Check sheet for the modelled part. Datum: model origin and axes. Units: mm. Face numbers are marked on the shaded views. Give positions to 0.01 mm unless a question says otherwise; leave off trailing zeros. Order: outer loops, then holes, each group sorted by start corner. A loop starts at its lowest first (then second) coordinate and runs counter-clockwise, first axis right, second up. Notation, with made-up numbers: M 6.25,73.5 L 32.25,73.5 A13 ccw 32.25,95.5 Z; hole C 17,50 d1. An arc over 180 degrees is marked long. Return JSON: item names as keys, results as strings. Group by question number.
from build123d import *

# Parameters (mm, degrees)
SKETCH_1_R          = 325
EXTRUDE_1_DEPTH     = 255
CUT_EXTRUDE_2_DEPTH = 255
CUT_EXTRUDE_3_DEPTH = 255
CUT_EXTRUDE_5_DEPTH = 255
CUT_EXTRUDE_6_DEPTH = 255


with BuildPart() as part:
    # 草图1 → 凸台-拉伸1 (new body)
    with BuildSketch(Plane.XY):
        Circle(SKETCH_1_R)
    extrude(amount=EXTRUDE_1_DEPTH)

    # 草图2 → 切除-拉伸2 (cut)
    with BuildSketch(Plane.XY):
        with BuildLine():
            Line((51.961524227, 30), (250, 30))
            ThreePointArc((250, 30), (185.563491861, 185.563491861), (30, 250))
            Line((30, 250), (30, 51.961524227))
            ThreePointArc((30, 51.961524227), (42.426406871, 42.426406871), (51.961524227, 30))
        make_face()
    extrude(amount=CUT_EXTRUDE_2_DEPTH, mode=Mode.SUBTRACT)

    # 草图3 → 切除-拉伸3 (cut)
    with BuildSketch(Plane.XY):
        with BuildLine():
            Line((-30, 250), (-30, 51.961524227))
            ThreePointArc((-30, 51.961524227), (-42.426406871, 42.426406871), (-51.961524227, 30))
            Line((-51.961524227, 30), (-250, 30))
            ThreePointArc((-250, 30), (-185.563491861, 185.563491861), (-30, 250))
        make_face()
    extrude(amount=CUT_EXTRUDE_3_DEPTH, mode=Mode.SUBTRACT)

    # 草图7 → 切除-拉伸5 (cut)
    with BuildSketch(Plane.XY):
        with BuildLine():
            Line((-30, -51.961524227), (-30, -250))
            ThreePointArc((-30, -250), (-185.563491861, -185.563491861), (-250, -30))
            Line((-250, -30), (-51.961524227, -30))
            ThreePointArc((-51.961524227, -30), (-42.426406871, -42.426406871), (-30, -51.961524227))
        make_face()
    extrude(amount=CUT_EXTRUDE_5_DEPTH, mode=Mode.SUBTRACT)

    # 草图8 → 切除-拉伸6 (cut)
    with BuildSketch(Plane.XY):
        with BuildLine():
            Line((30, -30), (30, -250))
            ThreePointArc((30, -250), (185.563491861, -185.563491861), (250, -30))
            Line((250, -30), (30, -30))
        make_face()
    extrude(amount=CUT_EXTRUDE_6_DEPTH, mode=Mode.SUBTRACT)


solid = part.part
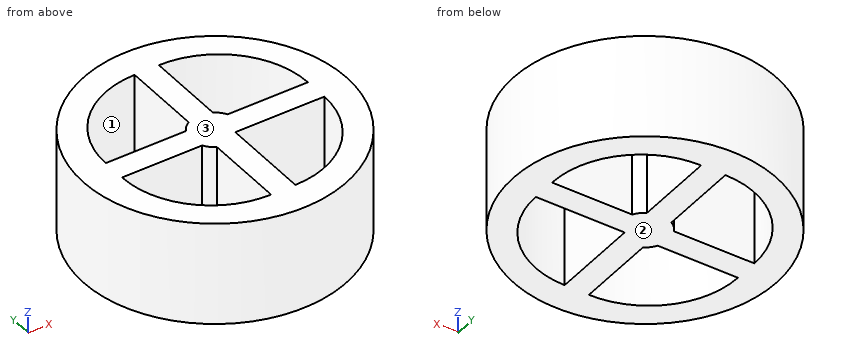
1) Sectioned sample at D-D on x = 266. Record the boundary of the cut face in (y, z).
2) Sectioned sample at A-A on y = -122.5. Record the boundary of the cut face in (x, z), then the cut area to 3 significant figures.
3) Release check for a two-part mould opening along Z. For the marked faces 1, 2 and 3 record: released by +Z, released by -Z, zero draft, split by the parting line, or undercut.
4) Sectioned sample at B-B on z = 91. Record the boundary of the cut face in (x, y), then the cut area to 3 significant figures.
5) Depth check by flat-ended pin: P1, Ø10, axis at x = -81, z = 30.5, coming from the -Y side; P2, Ø4, axis at x = 24, z = 84.5, coming from the -Y side; P3, Ø1.5, axis at y = 70, z = 72.5, coming from the +X side. Enter the tip coordinate at first touch or a pass-through.
6) Material ranges on line 1 along X through (y, z) = (-168.5, 104.5); line 2 along Y through (x, z) = (205, 216.5); line 3 along X through (y, z) = (-165, 18), recorded low to high.
7) Sectioned sample at C-C on x = 112.5. Record the boundary of the cut face in (y, z), then the cut area to 3 significant figures.
Reply:
{
 "1": {"outline": "M -186.73,0 L 186.73,0 L 186.73,255 L -186.73,255 Z"},
 "2": {"outline": "M -301.03,0 L -229.61,0 L -229.61,255 L -301.03,255 Z; M -30,0 L 30,0 L 30,255 L -30,255 Z; M 229.61,0 L 301.03,0 L 301.03,255 L 229.61,255 Z", "area": "51,700 mm^2"},
 "3": {"face 1": "zero draft", "face 2": "released by -Z", "face 3": "released by +Z"},
 "4": {"outline": "C 0,0 d650; hole M -250,-30 A220 ccw -30,-250 L -30,-51.96 A60 cw -51.96,-30 Z; hole M -250,30 L -51.96,30 A60 cw -30,51.96 L -30,250 A220 ccw Z; hole M 30,-250 A220 ccw 250,-30 L 30,-30 Z; hole M 30,51.96 A60 cw 51.96,30 L 250,30 A220 ccw 30,250 Z", "area": "181,000 mm^2"},
 "5": {"P1": "y = -315.99", "P2": "y = -324.25", "P3": "x = 317.54"},
 "6": {"line 1": "-277.91 to -200.93, -30 to 30, 200.93 to 277.91", "line 2": "-252.19 to -163.32, -30 to 30, 163.32 to 252.19", "line 3": "-280 to -203.71, -30 to 30, 203.71 to 280"},
 "7": {"outline": "M -304.91,0 L -233.95,0 L -233.95,255 L -304.91,255 Z; M -30,0 L 30,0 L 30,255 L -30,255 Z; M 233.95,0 L 304.91,0 L 304.91,255 L 233.95,255 Z", "area": "51,500 mm^2"}
}
